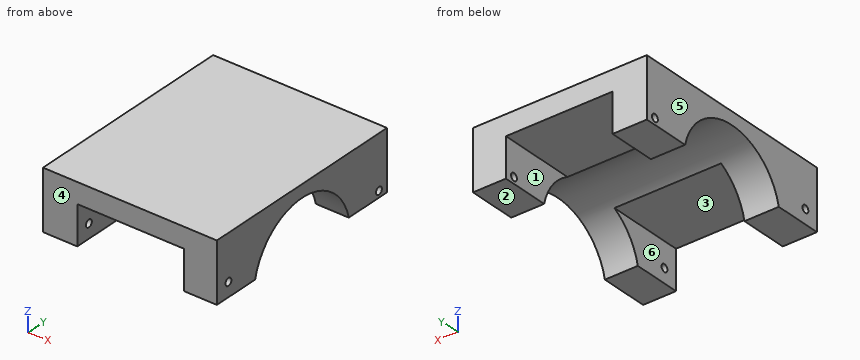
from build123d import *

# Parameters (mm, degrees)
F0_W     = 112.1267676353
F0_H     = 38.257420063
F1_DEPTH = 137.870118022
F2_W     = 68.7767341733
F2_H     = 25.1477137208
F3_DEPTH = 137.871118022
F4_R     = 2.38125
F5_DEPTH = 112.1277676353
F6_R     = 2.38125
F7_DEPTH = 112.1277676353
F9_DEPTH = 112.1277676353


with BuildPart() as f1:
    # F0 (on Front) → F1 (new body)
    with BuildSketch(Plane.XZ):
        with Locations((-1.3227313757, 19.1287100315)):
            Rectangle(F0_W, F0_H)
    extrude(amount=F1_DEPTH)

    # F2 (on face) → F3 (cut, through all)
    with BuildSketch(Plane.XZ.offset(137.870118022)):
        with Locations((-0.8782893419, 12.5738568604)):
            Rectangle(F2_W, F2_H)
    extrude(amount=-F3_DEPTH, mode=Mode.SUBTRACT)

    # F4 (on face) → F5 (cut, through all)
    with BuildSketch(Plane.YZ.offset(54.740652442)):
        with Locations((-128.4904330969, 9.1332495213)):
            Circle(F4_R)
    extrude(amount=-F5_DEPTH, mode=Mode.SUBTRACT)

    # F6 (on face) → F7 (cut, through all)
    with BuildSketch(Plane.YZ.offset(54.740652442)):
        with Locations((-6.499979645, 4.1290447116)):
            Circle(F6_R)
    extrude(amount=-F7_DEPTH, mode=Mode.SUBTRACT)

    # F8 (on face) → F9 (cut, through all)
    with BuildSketch(Plane.YZ.offset(54.740652442)):
        with BuildLine():
            Line((-106.8989974441, 0), (-30.9711205779, 0))
            ThreePointArc((-30.9711205779, 0), (-68.935059011, 30.0939472481), (-106.8989974441, 0))
        make_face()
    extrude(amount=-F9_DEPTH, mode=Mode.SUBTRACT)


solid = f1.part
Work out the finished part from the listing and answer in its coordinate system (mm). Face numbers are marked on the shaded views. A direction names the side the tool comes from. Round coordinates to 2 decimals unless told otherwise and drop trailing zeros. Write each loop counter-clockwise with the first axis right and the second up, starting at its lowest first coordinate (ties: lowest second). Pieces come first, ordered by that corner, then holes. Notation, with made-up numbers: (49.5, 13.25) - (86.5, 13.25) arc R11 cw to (86.5, 23.25) - close; hole circle Ø8 at (74.25, 83). An arc over 180 degrees is marked (long way). Answer in a Markdown table with one row per item. Add a question column.
1. A cutting plane is placed at A-A, the plane z = 22. Determine the outline of the cut face in (x, y), and give its area (3 significant figures).
2. A cutting plane is placed at D-D, the plane x = 21. Determine the outline of the cut face in (y, z).
3. The mould has two halves that part along X. Classify the marked faces 3, 4, 5 and 6: +X half, -X half, draft (parallel to the pull), parting line (faces both ways), or undercut.
4. A cutting plane is placed at B-B, the plane x = 44.5. Determine the outline of the cut face in (y, z).
5. For the marked faces 1 and 2, determine the directions among +Z, -Z, +X, -X, +Y, -Y from which every point of the face is accessible in a straight line to the end or side of a thin tool.
6. Find the intervals of material crossed by line 1 along X through (y, z) = (-106, 12.5); line 2 along Z through (x, y) = (-3, -37.5); line 3 along Y through (x, z) = (-36, 3.5), in increasing order. Write a range as from..to.
7. Given pin 1 (3 mm diameter, centred on y = -6.5, z = 4.13, fed in from -X); pin 2 (8 mm diameter, centred on x = -11.5, y = -78.5, fed in from -Z); pin 3 (25 mm diameter, centred on x = -2.5, y = -106.5, fed in from -Z), each flat-ended and moving along its own axis, determine where each tip first touches the part or whether it passes through.
8. A cutting plane is placed at C-C, the plane y = -123.5. Determine the outline of the cut face in (x, z), and give its area (3 significant figures).
Worked out:
| question | item | result |
|---|---|---|
| 1 | outline | (-57.39, -137.87) - (-35.27, -137.87) - (-35.27, -92.72) - (-57.39, -92.72) - close; (-57.39, -45.15) - (-35.27, -45.15) - (-35.27, 0) - (-57.39, 0) - close; (33.51, -137.87) - (54.74, -137.87) - (54.74, -92.72) - (33.51, -92.72) - close; (33.51, -45.15) - (54.74, -45.15) - (54.74, 0) - (33.51, 0) - close |
| 1 | area | 3,910 mm^2 |
| 2 | outline | (-137.87, 25.15) - (-87.94, 25.15) arc R38.99 cw to (-49.93, 25.15) - (0, 25.15) - (0, 38.26) - (-137.87, 38.26) - close |
| 3 | face 3 | undercut |
| 3 | face 4 | draft |
| 3 | face 5 | -X half |
| 3 | face 6 | undercut |
| 4 | outline | (-137.87, 0) - (-106.9, 0) arc R38.99 cw to (-30.97, 0) - (0, 0) - (0, 38.26) - (-137.87, 38.26) - close; hole circle Ø4.76 at (-128.49, 9.13); hole circle Ø4.76 at (-6.5, 4.13) |
| 5 | face 1 | -Z, +Y, -Y |
| 5 | face 2 | -Z, +X, -X, +Y, -Y |
| 6 | line 1 | -57.39..-35.27, 33.51..54.74 |
| 6 | line 2 | 25.15..38.26 |
| 6 | line 3 | -137.87..-105.9, -31.97..-8.8, -4.2..0 |
| 7 | pin 1 | through |
| 7 | pin 2 | z = 27.66 |
| 7 | pin 3 | z = 25.15 |
| 8 | outline | (-57.39, 0) - (-35.27, 0) - (-35.27, 25.15) - (33.51, 25.15) - (33.51, 0) - (54.74, 0) - (54.74, 38.26) - (-57.39, 38.26) - close |
| 8 | area | 2,560 mm^2 |
